The model under review builds one solid part; all positions refer to its coordinate system, in mm. A direction names the side the tool comes from. Coordinates: 2 decimals unless noted, no trailing zeros. Loops run counter-clockwise (first coordinate to the right, second up) from the corner with the lowest first, then second, coordinate; pieces in that order, holes last. Notation, with made-up numbers: M 57,-16.75 L 85,-16.75 A24 cw 85,19.25 Z; hole C 50,-33 d6. An arc over 180 degrees is marked long. Return JSON: item names as keys, results as strings.
```python
from build123d import *

# Parameters (mm, degrees)
SKETCH_1_R             = 6
EXTRUDE_1_DEPTH        = 15
SKETCH_3_R             = 4
EXTRUDE_3_DEPTH        = 1
FILLET_2_R             = 0.5
EXTRUDE_START          = 7.5
SKETCH_4_W             = 4
SKETCH_4_H             = 1.5
EXTRUDE_4_DEPTH        = 6
F_1_0MM_1_D            = 1
FILLET_3_R             = 0.2
SKETCH_7_R             = 1.5
CUT_EXTRUDE_1_DEPTH    = 20.006577809
HOLE_WIZARD_M2_1_D     = 0.6
HOLE_WIZARD_M2_1_DEPTH = 2.5
HOLE_WIZARD_M2_1_TIP   = 0.180258186


with BuildPart() as part:
    # 草圖1 → 填料-伸長1 (new body)
    with BuildSketch(Plane.XY):
        Circle(SKETCH_1_R)
    extrude(amount=EXTRUDE_1_DEPTH)

    # 草圖3 → 填料-伸長3 (add)
    with BuildSketch(Plane(origin=(0, 0, 0), x_dir=(-1, 0, 0), z_dir=(0, 0, -1))):
        Circle(SKETCH_3_R)
    extrude(amount=EXTRUDE_3_DEPTH)

    # 圓角2
    fillet_2_edges = [part.edges().sort_by_distance(p)[0] for p in [
        (-6, 0, 0),
        (-6, 0, 15),
    ]]
    fillet(fillet_2_edges, radius=FILLET_2_R)

    # 草圖4 → 填料-伸長4 (add, symmetric)
    with BuildSketch(Plane.XY.offset(EXTRUDE_START)):
        with Locations((5.5, -6.25)):
            Rectangle(SKETCH_4_W, SKETCH_4_H)
        with BuildLine():
            Line((2.5, -5.454356057), (3.5, -7))
            Line((3.5, -7), (3.5, -5.5))
            Line((3.5, -5.5), (5.361902647, -5.5))
            ThreePointArc((5.361902647, -5.5), (4.45557568, -4.922577127), (4.595916555, -3.857142857))
            ThreePointArc((4.595916555, -3.857142857), (3.636726611, -4.772234231), (2.5, -5.454356057))
        make_face()
    extrude_4 = extrude(amount=EXTRUDE_4_DEPTH, both=True)

    # Ø1.0mm 定位孔1 (through all)
    with Locations(Plane(origin=(0, -5.5, 0), x_dir=(1, 0, 0), z_dir=(0, 1, 0))):
        with Locations((6.7, -3.5), (6.7, -11.5)):
            f_1_0mm_1 = Hole(F_1_0MM_1_D / 2)

    # 鏡射1: 填料-伸長4, Ø1.0mm 定位孔1 across plane
    add(extrude_4.mirror(Plane(origin=(0, 0, 0), x_dir=(0, 0, 1), z_dir=(1, 0, 0))))
    add(f_1_0mm_1.mirror(Plane(origin=(0, 0, 0), x_dir=(0, 0, 1), z_dir=(1, 0, 0))), mode=Mode.SUBTRACT)

    # 圓角3
    fillet_3_edges = [part.edges().sort_by_distance(p)[0] for p in [
        (4, 0, 0),
        (4, 0, -1),
    ]]
    fillet(fillet_3_edges, radius=FILLET_3_R)

    # 草圖7 → 除料-伸長1 (cut, through all)
    with BuildSketch(Plane.XY.offset(15)):
        Circle(SKETCH_7_R)
    extrude(amount=-CUT_EXTRUDE_1_DEPTH, mode=Mode.SUBTRACT)

    # M2 螺紋孔1
    with Locations(Plane.XY.offset(15)):
        with Locations((0, 4.5), (3.897114317, -2.25), (-3.897114317, -2.25)):
            Hole(HOLE_WIZARD_M2_1_D / 2, depth=HOLE_WIZARD_M2_1_DEPTH)
            with Locations((0, 0, -(HOLE_WIZARD_M2_1_DEPTH + HOLE_WIZARD_M2_1_TIP / 2))):  # 118° drill point
                Cone(0, HOLE_WIZARD_M2_1_D / 2, HOLE_WIZARD_M2_1_TIP, mode=Mode.SUBTRACT)


solid = part.part
```
1. The part is to be moulded in two halves that separate along X. For faces 6 (the face through (2.993, -6.216, 7.584)), 7 (the face through (1.1, 1.3, 15)), 8 (the face through (4.462, -4.937, 7.584)), say which applies: released by +X, released by -X, zero draft, split by the parting line, or undercut.
Check values:
{"face 6": "undercut", "face 7": "zero draft", "face 8": "released by +X"}
2. Insertion check: pin 1 Ø0.9 at (x, y) = (-4.5, -5) entering from +Z; pin 2 Ø2.5 at (x, y) = (-4, -5) entering from -Z; pin 3 Ø1.6 at (x, y) = (4, -5) entering from +Z. Each pin has a flat end and moves straight along its axis. Give the tip position at first contact, or say it passes through.
Check values:
{"pin 1": "z = 13.5", "pin 2": "z = 0", "pin 3": "z = 14.99"}
3. Add section A-A on x = -6.7. Give the boundary of the cut face in (y, z).
Check values:
{"outline": "M -7,1.5 L -5.5,1.5 L -5.5,3 L -7,3 Z; M -7,4 L -5.5,4 L -5.5,11 L -7,11 Z; M -7,12 L -5.5,12 L -5.5,13.5 L -7,13.5 Z"}
4. Add section B-B on z = 3.5. Give the boundary of the cut face in (x, y).
Check values:
{"outline": "M -7.5,-7 L -7.2,-7 L -7.2,-5.5 L -7.5,-5.5 Z; M -6.2,-7 L -3.5,-7 L -2.5,-5.45 A6 ccw 2.5,-5.45 L 3.5,-7 L 6.2,-7 L 6.2,-5.5 L 5.36,-5.5 A1 cw 4.6,-3.86 A6 ccw long -4.6,-3.86 A1 cw -5.36,-5.5 L -6.2,-5.5 Z; M 7.2,-7 L 7.5,-7 L 7.5,-5.5 L 7.2,-5.5 Z; hole C 0,0 d3"}
5. Add section C-C on z = 10.25. Give the boundary of the cut face in (x, y), plus the area to 3 significant figures.
Check values:
{"outline": "M -7.5,-7 L -3.5,-7 L -2.5,-5.45 A6 ccw 2.5,-5.45 L 3.5,-7 L 7.5,-7 L 7.5,-5.5 L 5.36,-5.5 A1 cw 4.6,-3.86 A6 ccw long -4.6,-3.86 A1 cw -5.36,-5.5 L -7.5,-5.5 Z; hole C 0,0 d3", "area": "122 mm²"}
6. To check wall thickness, follow line 1 (Z direction, x = 6.7, y = -5.85); line 2 (X direction, y = -2.25, z = 13.85); line 3 (Z direction, x = 0.5, y = 4.75). State the ranges of each line that lie inside material, in increasing order.
Check values:
{"line 1": "1.5 to 3, 4 to 11, 12 to 13.5", "line 2": "-5.56 to -4.2, -3.6 to 3.6, 4.2 to 5.56", "line 3": "0 to 15"}
7. Machinability: for faces 1 (the face through (5, -6, 1.5)), 2 (the face through (-5, -6, 13.5)), 3 (the face through (-4, -2, 0)), 4 (the face through (5, -6, 13.5)), 5 (the face through (-2.993, -6.216, 7.584)), which of the approach directions +Z, -Z, +X, -X, +Y, -Y give a long, thin tool a straight path to every point of the face, cutting with its end or side? Answer none if there is none.
Check values:
{"face 1": "-Z, +X, -Y", "face 2": "+Z, -X, -Y", "face 3": "-Z", "face 4": "+Z, +X, -Y", "face 5": "+Z, -Z, -Y"}
